from build123d import *

# Parameters (mm, degrees)
SKETCH1_R           = 28.575
BOSS_EXTRUDE1_DEPTH = 6.35
SKETCH2_R           = 14.2875
BOSS_EXTRUDE2_DEPTH = 12.7
CUT_EXTRUDE1_DEPTH  = 20.05
SKETCH4_R           = 2
CUT_EXTRUDE2_DEPTH  = 7.35
FILLET1_R           = 1


with BuildPart() as part:
    # Sketch1 → Boss-Extrude1 (new body)
    with BuildSketch(Plane.XY):
        Circle(SKETCH1_R)
    extrude(amount=BOSS_EXTRUDE1_DEPTH)

    # Sketch2 → Boss-Extrude2 (add)
    with BuildSketch(Plane.XY.offset(6.35)):
        Circle(SKETCH2_R)
    extrude(amount=BOSS_EXTRUDE2_DEPTH)

    # Sketch3 → Cut-Extrude1 (cut, through all)
    with BuildSketch(Plane.XY.offset(19.05)):
        Polygon((7.332348419, 0), (3.666174209, 6.35), (-3.666174209, 6.35), (-7.332348419, 0), (-3.666174209, -6.35), (3.666174209, -6.35), align=None)
    extrude(amount=-CUT_EXTRUDE1_DEPTH, mode=Mode.SUBTRACT)

    # Sketch4 → Cut-Extrude2 (cut, through all)
    with BuildSketch(Plane.XY.offset(6.35)):
        with Locations((25.4, 0)):
            Circle(SKETCH4_R)
        with Locations((12.7, -21.997045256)):
            Circle(SKETCH4_R)
        with Locations((-12.7, -21.997045256)):
            Circle(SKETCH4_R)
        with Locations((-25.4, 0)):
            Circle(SKETCH4_R)
        with Locations((-12.7, 21.997045256)):
            Circle(SKETCH4_R)
        with Locations((12.7, 21.997045256)):
            Circle(SKETCH4_R)
    extrude(amount=-CUT_EXTRUDE2_DEPTH, mode=Mode.SUBTRACT)

    # Fillet1
    fillet1_edges = [part.edges().sort_by_distance(p)[0] for p in [
        (5.499261314, -3.175, 19.05),
        (5.499261314, 3.175, 19.05),
        (0, 6.35, 19.05),
        (-5.499261314, 3.175, 19.05),
        (-5.499261314, -3.175, 19.05),
        (0, -6.35, 19.05),
    ]]
    fillet(fillet1_edges, radius=FILLET1_R)


solid = part.part
Work out the finished part from the listing and answer in its coordinate system (mm). A direction names the side the tool comes from. Round coordinates to 2 decimals unless told otherwise and drop trailing zeros. Write each loop counter-clockwise with the first axis right and the second up, starting at its lowest first coordinate (ties: lowest second). Pieces come first, ordered by that corner, then holes. Notation, with made-up numbers: (62, -20.75) - (120, -20.75) arc R22 cw to (120, -7.75) - close; hole circle Ø7 at (1, 21). An arc over 180 degrees is marked (long way). Answer in a Markdown table with one row per item. Add a question column.
1. For faces 4 (the flat face through (0, 7, 0)), 5 (the flat face through (5.525, 3.131, 9.151)), 6 (the cylindrical face through (-5.776, 3.266, 18.749)), determine the directions among +Z, -Z, +X, -X, +Y, -Y from which every point of the face is accessible in a straight line to the end or side of a thin tool.
2. Find the intervals of material crossed by line 1 along Y through (x, z) = (12.7, 3); line 2 along Z through (x, y) = (-21, 4.5); line 3 along Y through (x, z) = (-12, 2.25), in increasing order. Write a range as from..to.
3. A cutting plane is placed at C-C, the plane x = 12.7. Determine the outline of the cut face in (y, z), and give its area (3 significant figures).
4. Given pin 1 (10 mm diameter, centred on x = 13.5, z = 16, fed in from -Y); pin 2 (2.5 mm diameter, centred on x = 25.4, y = 0, fed in from +Z); pin 3 (5 mm diameter, centred on x = -7, z = 2.5, fed in from -Y); pin 4 (2 mm diameter, centred on x = 17, y = 14, fed in from +Z), each flat-ended and moving along its own axis, determine where each tip first touches the part or whether it passes through.
5. A cutting plane is placed at D-D, the plane z = 2.25. Determine the outline of the cut face in (x, y) (3 decimals).
6. The mould has two halves that part along X. Classify faces 1 (the flat face through (0, 6.35, 9)), 2 (the flat face through (-13, 7, 6.35)), 3 (the cylindrical face through (-28.547, 1.256, 3.131)): +X half, -X half, draft (parallel to the pull), parting line (faces both ways), or undercut.
Worked out:
| question | item | result |
|---|---|---|
| 1 | face 4 | -Z, +X, -X, +Y, -Y |
| 1 | face 5 | +Z, -Z |
| 1 | face 6 | +Z |
| 2 | line 1 | -25.6..-24, -20..20, 24..25.6 |
| 2 | line 2 | 0..6.35 |
| 2 | line 3 | -25.93..-23.87, -20.12..20.12, 23.87..25.93 |
| 3 | outline | (-25.6, 0) - (-24, 0) - (-24, 6.35) - (-25.6, 6.35) - close; (-20, 0) - (20, 0) - (20, 6.35) - (6.55, 6.35) - (6.55, 19.05) - (-6.55, 19.05) - (-6.55, 6.35) - (-20, 6.35) - close; (24, 0) - (25.6, 0) - (25.6, 6.35) - (24, 6.35) - close |
| 3 | area | 441 mm^2 |
| 4 | pin 1 | y = -11.48 |
| 4 | pin 2 | through |
| 4 | pin 3 | y = -28.22 |
| 4 | pin 4 | z = 6.35 |
| 5 | outline | circle Ø57.15 at (0, 0); hole circle Ø4 at (-25.4, 0); hole circle Ø4 at (-12.7, -21.997); hole circle Ø4 at (-12.7, 21.997); hole (-7.332, 0) - (-3.666, -6.35) - (3.666, -6.35) - (7.332, 0) - (3.666, 6.35) - (-3.666, 6.35) - close; hole circle Ø4 at (12.7, -21.997); hole circle Ø4 at (12.7, 21.997); hole circle Ø4 at (25.4, 0) |
| 6 | face 1 | undercut |
| 6 | face 2 | draft |
| 6 | face 3 | parting line |
